Input: part model. Units: mm. Frame: model coordinates. Face numbers are marked on the shaded views. A direction names the side the tool comes from. Give positions to 0.01 mm unless a question says otherwise; leave off trailing zeros. Loops run counter-clockwise (first coordinate to the right, second up) from the corner with the lowest first, then second, coordinate; pieces in that order, holes last. Notation, with made-up numbers: (8, 45.5) -> (31, 45.5) arc R19 ccw to (31, 60.5) -> close; hole circle Ø10 at (81.5, -16.75). An arc over 180 degrees is marked (long way). Use CSV: the item, a comma, the result in double quotes.
```python
from build123d import *

# Parameters (mm, degrees)
SKETCH1_W                 = 40
SKETCH1_H                 = 9
BOSS_EXTRUDE1_DEPTH       = 4
F_8_CLEARANCE_HOLE1_D     = 4.4958
F_8_CLEARANCE_HOLE1_DEPTH = 17
F_8_CLEARANCE_HOLE1_TIP   = 1.350674586
SKETCH5_W                 = 2
SKETCH5_H                 = 9
BOSS_EXTRUDE2_DEPTH       = 5
BOSS_EXTRUDE2_DEPTH_BACK  = 9
SKETCH6_R                 = 1.5
CUT_EXTRUDE1_DEPTH        = 2


with BuildPart() as part:
    # Sketch1 → Boss-Extrude1 (new body)
    with BuildSketch(Plane(origin=(0, 0, 0), x_dir=(1, 0, 0), z_dir=(0, 1, 0))):
        with Locations((12.773632998, 0.813559322)):
            Rectangle(SKETCH1_W, SKETCH1_H)
    extrude(amount=BOSS_EXTRUDE1_DEPTH)

    # #8 Clearance Hole1
    with Locations(Plane(origin=(0.773632998, 4, -0.813559322), x_dir=(0, 0, 1), z_dir=(0, 1, 0))):
        with Locations((0, 0), (0, 24)):
            Hole(F_8_CLEARANCE_HOLE1_D / 2, depth=F_8_CLEARANCE_HOLE1_DEPTH)
            with Locations((0, 0, -(F_8_CLEARANCE_HOLE1_DEPTH + F_8_CLEARANCE_HOLE1_TIP / 2))):  # 118° drill point
                Cone(0, F_8_CLEARANCE_HOLE1_D / 2, F_8_CLEARANCE_HOLE1_TIP, mode=Mode.SUBTRACT)

    # Sketch5 → Boss-Extrude2 (add, two sides)
    with BuildSketch(Plane(origin=(0, 4, 0), x_dir=(1, 0, 0), z_dir=(0, 1, 0))) as boss_extrude2_sk:
        with Locations((13.773632998, 0.813559322)):
            Rectangle(SKETCH5_W, SKETCH5_H)
    extrude(amount=BOSS_EXTRUDE2_DEPTH)
    extrude(boss_extrude2_sk.sketch, amount=-BOSS_EXTRUDE2_DEPTH_BACK)

    # Sketch6 → Cut-Extrude1 (cut)
    with BuildSketch(Plane.ZY.offset(-12.773632998)):
        with Locations((-0.813559322, 6.5)):
            Circle(SKETCH6_R)
        with Locations((-0.813559322, -2.5)):
            Circle(SKETCH6_R)
    extrude(amount=-CUT_EXTRUDE1_DEPTH, mode=Mode.SUBTRACT)


solid = part.part
```
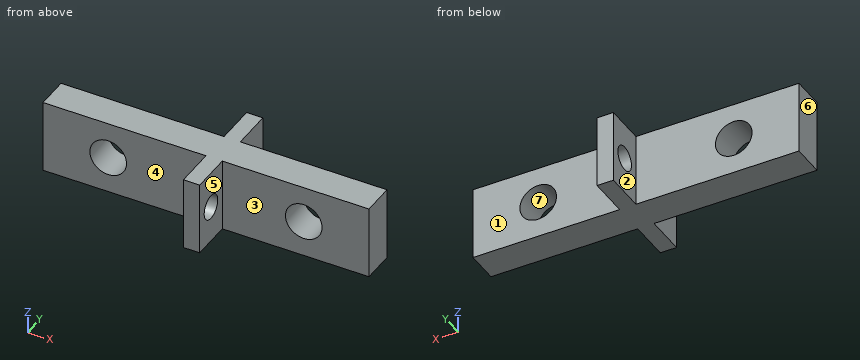
1) Mould query, pull axis X, two halves, no side actions, for the marked faces 5, 6 and 7. Classes: pulls with the +X half, pulls with the -X half, needs draft (parallel to the pull), parting line crosses it, or undercut.
From the geometry:
face 5,"pulls with the +X half"
face 6,"pulls with the -X half"
face 7,"undercut"
2) Section query C-C (y = 3.5). Return loops of the section in (x, z).
From the geometry:
outline,"(-7.23, -5.31) -> (32.77, -5.31) -> (32.77, 3.69) -> (-7.23, 3.69) -> close; hole circle Ø4.5 at (0.77, -0.81); hole circle Ø4.5 at (24.77, -0.81)"
3) Contact query for flat-ended pins moving along their axis: pin 1 (1.5 mm diameter, centred on y = 6, z = -2.5, fed in from -X); pin 2 (1 mm diameter, centred on x = 26, z = -4.5, fed in from +Y). Output: stop coordinate, or through.
From the geometry:
pin 1,"stops at x = 12.77"
pin 2,"stops at y = 4"
4) Section query D-D (x = -5). Return loops of the section in (y, z).
From the geometry:
outline,"(0, -5.31) -> (4, -5.31) -> (4, 3.69) -> (0, 3.69) -> close"
5) Section query A-A (y = -2.5). Return loops of the section in (x, z), then the cut area to 3 significant figures.
From the geometry:
outline,"(12.77, -5.31) -> (14.77, -5.31) -> (14.77, -2.31) -> (12.77, -2.31) -> close; (12.77, 0.69) -> (14.77, 0.69) -> (14.77, 3.69) -> (12.77, 3.69) -> close"
area,"12.0 mm^2"
6) Section query B-B (z = 2). Return loops of the section in (x, y).
From the geometry:
outline,"(-7.23, 0) -> (12.77, 0) -> (12.77, -5) -> (14.77, -5) -> (14.77, 0) -> (32.77, 0) -> (32.77, 4) -> (14.77, 4) -> (14.77, 9) -> (12.77, 9) -> (12.77, 4) -> (-7.23, 4) -> close"
7) Ray query, line 1 (Y direction, x = 22.5, z = -2); line 2 (X direction, y = -0.75, z = 0); line 3 (X direction, y = 1.75, z = -0.25). Return the intervals inside material, ascending.
From the geometry:
line 1,"y = 0 to 4"
line 2,"x = 12.77 to 14.77"
line 3,"x = -7.23 to -1.4, 2.95 to 22.6, 26.95 to 32.77"
8) Reachability of the marked faces 1, 2, 3 and 4 from +Z, -Z, +X, -X, +Y, -Y: full face, straight path, thin tool, end or side. Return the list, or none.
From the geometry:
face 1,"+Z, -Z, +X, +Y"
face 2,"+Z, -Z, -X, +Y"
face 3,"+Z, -Z, +X, -Y"
face 4,"+Z, -Z, -X, -Y"
